Geometry check sheet. Reference: the model listing, model coordinates, mm. Give positions to 0.01 mm unless a question says otherwise; leave off trailing zeros. Loops run counter-clockwise (first coordinate to the right, second up) from the corner with the lowest first, then second, coordinate; pieces in that order, holes last. Notation, with made-up numbers: (82.25, 14) - (135.25, 14) arc R10 cw to (135.25, 27) - close; hole circle Ø8 at (14.5, 83.25). An arc over 180 degrees is marked (long way). Use a Markdown table: item, result. Add a question column.
1. Depth check by flat-ended pin: P1, Ø10, axis at y = -1, z = 17, coming from the -X side; P2, Ø10, axis at x = -9, z = 17.5, coming from the -Y side; P3, Ø2, axis at x = 5, z = 4, coming from the +Y side. Enter the tip coordinate at first touch or a pass-through.
2. Cross-section at C-C on z = 10.5. Enter the section's corners in (x, y).
3. Cross-section at D-D on x = 17. Enter the section's corners in (y, z).
4. Material ranges on L1, parallel to Y at x = 0, z = 9.75; L2, parallel to Z at x = 8, y = 4; L3, parallel to X at y = -1, z = 2.5, recorded low to high.
5. Cross-section at A-A on y = 0. Enter the section's corners in (x, z), and give its area (3 significant figures).
6. Draft check along X on faces 1 (the cylindrical face through (2.192, -4.214, 10.86)), 2 (the cylindrical face through (-3.746, 0.165, 10.353)), 3 (the flat face through (0, 5, 1)). Enter one of: pulls with the +X half, pulls with the -X half, needs draft (parallel to the pull), parting line crosses it, or undercut.
from build123d import *

# Parameters (mm, degrees)
SKETCH1_R               = 21
BOSS_EXTRUDE1_DEPTH     = 1
SKETCH2_R               = 4.75
BOSS_EXTRUDE2_DEPTH     = 20
CUT_EXTRUDE1_DEPTH      = 37.373066959
CUT_EXTRUDE1_DEPTH_BACK = 37.373066959
SKETCH3_R               = 3.75


with BuildPart() as part:
    # Sketch1 → Boss-Extrude1 (new body)
    with BuildSketch(Plane.XY):
        Circle(SKETCH1_R)
    extrude(amount=BOSS_EXTRUDE1_DEPTH)

    # Sketch2 → Boss-Extrude2 (add)
    with BuildSketch(Plane.XY.offset(1)):
        Circle(SKETCH2_R)
    extrude(amount=BOSS_EXTRUDE2_DEPTH)

    # Sketch3 → Cut-Extrude1 (cut, two sides: drawn at the far end of the back side and taken through both)
    with BuildSketch(Plane.XY.offset(21).offset(-CUT_EXTRUDE1_DEPTH_BACK)):
        Circle(SKETCH3_R)
    extrude(amount=CUT_EXTRUDE1_DEPTH + CUT_EXTRUDE1_DEPTH_BACK, mode=Mode.SUBTRACT)


solid = part.part
Values found:
| question | item | result |
|---|---|---|
| 1 | P1 | stops at x = -4.75 |
| 1 | P2 | stops at y = -2.56 |
| 1 | P3 | stops at y = 2.56 |
| 2 | outline | circle Ø9.5 at (0, 0); hole circle Ø7.5 at (0, 0) |
| 3 | outline | (-12.33, 0) - (12.33, 0) - (12.33, 1) - (-12.33, 1) - close |
| 4 | L1 | y = -4.75 to -3.75, 3.75 to 4.75 |
| 4 | L2 | z = 0 to 1 |
| 4 | L3 | x = -4.64 to -3.61, 3.61 to 4.64 |
| 5 | outline | (-21, 0) - (-3.75, 0) - (-3.75, 21) - (-4.75, 21) - (-4.75, 1) - (-21, 1) - close; (3.75, 0) - (21, 0) - (21, 1) - (4.75, 1) - (4.75, 21) - (3.75, 21) - close |
| 5 | area | 74.5 mm2 |
| 6 | face 1 | parting line crosses it |
| 6 | face 2 | undercut |
| 6 | face 3 | needs draft |
